Verification items for the finished model (mm, model axes). A direction names the side the tool comes from. Round coordinates to 2 decimals unless told otherwise and drop trailing zeros. Order: outer loops, then holes, each group sorted by start corner. A loop starts at its lowest first (then second) coordinate and runs counter-clockwise, first axis right, second up. Notation, with made-up numbers: M 86.25,37 L 119.25,37 A10 ccw 119.25,43 Z; hole C 39,-27 d6. An arc over 180 degrees is marked long. Write item = value, one per line. Start each with the question number.
from build123d import *

# Parameters (mm, degrees)
F0_W     = 40
F0_H     = 10
F1_DEPTH = 25


with BuildPart() as f1:
    # F0 (on Front) → F1 (new body)
    with BuildSketch(Plane.XZ):
        Polygon((0, -20), (0, 0), (-40, 0), (-42, 0), (-42, -20), align=None)
        with Locations((-20, 5)):
            Rectangle(F0_W, F0_H)
        Polygon((-40, 10), (0, 10), (0, 60), (-50, 60), (-50, 10), align=None)
        Polygon((0, -50), (0, -20), (-42, -20), (-43, -20), (-43, -50), align=None)
    extrude(amount=F1_DEPTH)


solid = f1.part
1) Access from +Z, -Z, +X, -X, +Y, -Y to the whole of each face (thin tool, end or side, straight path). Record for faces 4 (the flat face through (-25, 0, 6)), 5 (the flat face through (-43, -12, -35)), 6 (the flat face through (-42, -12, -10)).
2) Cross-section at A-A, the plane y = -19. Enter the section's corners in (x, z), then the cut area to 3 significant figures.
3) Gauge pin test, flat ends, axial feed: P1, Ø6, axis at x = -34.5, z = 39, coming from the +Y side; P2, Ø5, axis at y = -7.5, z = 7, coming from the -X side; P3, Ø6, axis at y = -9.5, z = -6, coming from the -X side. Record the tip position at first contact, or that the pin passes through.
4) Cross-section at B-B, the plane x = -46. Enter the section's corners in (y, z).
5) Release check for a two-part mould opening along Z. For faces 1 (the flat face through (-41, -12, 0)), 2 (the flat face through (-25, -12, 60)), 3 (the flat face through (-25, -25, 6)) record: pulls with the +Z half, pulls with the -Z half, needs draft (parallel to the pull), parting line crosses it, or undercut.
6) Cross-section at C-C, the plane z = -9. Enter the section's corners in (x, y).
7) Scan lines: probe 1 along Z at (x, y) = (-48, -3.5); probe 2 along X at (y, z) = (-7, -41.5). Record each from-to range of solid material in increasing order.
Geometry results:
q1.face_4 = +Z, -Z, +X, -X, +Y
q1.face_5 = -Z, -X, +Y, -Y
q1.face_6 = -X, +Y, -Y
q2.outline = M -50,10 L -40,10 L -40,0 L -42,0 L -42,-20 L -43,-20 L -43,-50 L 0,-50 L 0,60 L -50,60 Z
q2.area = 5,030 mm^2
q3.P1 = 0
q3.P2 = -40
q3.P3 = -42
q4.outline = M -25,10 L 0,10 L 0,60 L -25,60 Z
q5.face_1 = undercut
q5.face_2 = pulls with the +Z half
q5.face_3 = needs draft
q6.outline = M -42,-25 L 0,-25 L 0,0 L -42,0 Z
q7.probe_1 = 10 to 60
q7.probe_2 = -43 to 0
